Read the model definition and answer for the solid it produces. Units are mm, in the model's axes. A direction names the side the tool comes from. Round coordinates to 2 decimals unless told otherwise and drop trailing zeros. Order: outer loops, then holes, each group sorted by start corner. A loop starts at its lowest first (then second) coordinate and runs counter-clockwise, first axis right, second up. Notation, with made-up numbers: (-34, 73.25) - (-20, 73.25) arc R9 cw to (-20, 80.25) - close; hole circle Ø10 at (-26, 64). An arc over 180 degrees is marked (long way). Answer as a JSON object with one key per item and string values. Group by question number.
Q1. A cutting plane is placed at D-D on z = -27.5. Determine the outline of the cut face in (x, y), and give its area (3 significant figures).
Q2. A tool of negligible diameter and unlimited length cuts with its end or side. For faces 4 (the flat face through (0, 47, -12.5)), 5 (the cylindrical face through (1.352, 22.185, -4.292)), 6 (the flat face through (-12.5, 47, 0)), 7 (the flat face through (3, 51, 0)), from which of +Z, -Z, +X, -X, +Y, -Y can it reach the whole face along a straight path? Write none if from no direction.
Q3. The mould has two halves that part along X. Classify faces 1 (the cylindrical face through (1.43, 21.76, 32.03)), 2 (the flat face through (12.5, 47, 0)), 3 (the flat face through (-9, 0, -1)): pulls with the +X half, pulls with the -X half, needs draft (parallel to the pull), parting line crosses it, or undercut.
Q4. A cutting plane is placed at B-B on y = 42. Determine the outline of the cut face in (x, z), and give its area (3 significant figures).
Q5. A cutting plane is placed at A-A on z = -13.75. Determine the outline of the cut face in (x, y), and give its area (3 significant figures).
Q6. Consider line 1 (Z direction, x = 2.5, y = 37); line 2 (X direction, y = 1.45, z = 13.75); line 3 (Z direction, x = 24, y = 13). Determine where each line is inside the solid, lowest interval first.
Q7. Given pin 1 Ø5 at (x, z) = (-1.5, 27) entering from +Y; pin 2 Ø14.5 at (x, z) = (0, 0) entering from +Y; pin 3 Ø2 at (y, z) = (13.5, -31) entering from +X; pin 4 Ø12 at (y, z) = (31, 9.5) entering from -X, each flat-ended and moving along its own axis, determine where each tip first touches the part or whether it passes through.
Q8. A cutting plane is placed at C-C on x = 0. Count the separate pieces of the cut face and the enclosed holes in it, and give its area (3 significant figures).
```python
from build123d import *

# Parameters (mm, degrees)
SKETCH1_R             = 41.5
MAIN_PLATE_DEPTH      = 40
SKETCH2_R             = 2.05
CUT_EXTRUDE_G27_DEPTH = 72.024643611
SKETCH5_R             = 4.75
G27_SCREW_HEADS_DEPTH = 37
SKETCH6_W             = 25
SKETCH6_H             = 25
BOSS_EXTRUDE1_DEPTH   = 15
SKETCH8_R             = 4.5
CUT_EXTRUDE1_DEPTH    = 45
SKETCH10_R            = 2.5
CUT_EXTRUDE3_DEPTH    = 81.4332021
CUT_EXTRUDE4_DEPTH    = 4


with BuildPart() as part:
    # Sketch1 → Main Plate (new body)
    with BuildSketch(Plane(origin=(0, 0, 0), x_dir=(1, 0, 0), z_dir=(0, 1, 0))):
        with Locations(Location((0, 0, 0), (0, 0, 270))):
            Circle(SKETCH1_R)
    extrude(amount=MAIN_PLATE_DEPTH)

    # Sketch2 → Cut-Extrude G27 (cut, through all)
    with BuildSketch(Plane(origin=(0, 40, 0), x_dir=(1, 0, 0), z_dir=(0, 1, 0))):
        with Locations(Location((0, 27.5, 0), (0, 0, 270))):
            Circle(SKETCH2_R)
        with Locations(Location((23.815698604, 13.75, 0), (0, 0, 270))):
            Circle(SKETCH2_R)
        with Locations(Location((23.815698604, -13.75, 0), (0, 0, 270))):
            Circle(SKETCH2_R)
        with Locations(Location((0, -27.5, 0), (0, 0, 270))):
            Circle(SKETCH2_R)
        with Locations(Location((-23.815698604, -13.75, 0), (0, 0, 270))):
            Circle(SKETCH2_R)
        with Locations(Location((-23.815698604, 13.75, 0), (0, 0, 270))):
            Circle(SKETCH2_R)
    extrude(amount=-CUT_EXTRUDE_G27_DEPTH, mode=Mode.SUBTRACT)

    # Sketch5 → G27 Screw Heads (cut)
    with BuildSketch(Plane(origin=(0, 40, 0), x_dir=(1, 0, 0), z_dir=(0, 1, 0))):
        with Locations(Location((0, 27.5, 0), (0, 0, 270))):
            Circle(SKETCH5_R)
        with Locations(Location((23.815698604, 13.75, 0), (0, 0, 270))):
            Circle(SKETCH5_R)
        with Locations(Location((23.815698604, -13.75, 0), (0, 0, 270))):
            Circle(SKETCH5_R)
        with Locations(Location((0, -27.5, 0), (0, 0, 270))):
            Circle(SKETCH5_R)
        with Locations(Location((-23.815698604, -13.75, 0), (0, 0, 270))):
            Circle(SKETCH5_R)
        with Locations(Location((-23.815698604, 13.75, 0), (0, 0, 270))):
            Circle(SKETCH5_R)
    extrude(amount=-G27_SCREW_HEADS_DEPTH, mode=Mode.SUBTRACT)

    # Sketch6 → Boss-Extrude1 (add)
    with BuildSketch(Plane(origin=(0, 40, 0), x_dir=(1, 0, 0), z_dir=(0, 1, 0))):
        Rectangle(SKETCH6_W, SKETCH6_H)
    extrude(amount=BOSS_EXTRUDE1_DEPTH)

    # Sketch8 → Cut-Extrude1 (cut)
    with BuildSketch(Plane.XZ):
        with Locations(Location((0, 0, 0), (0, 0, 270))):
            Circle(SKETCH8_R)
    extrude(amount=-CUT_EXTRUDE1_DEPTH, mode=Mode.SUBTRACT)

    # Cut-Extrude2 cone 1 section (through the dimple's axis) → Cut-Extrude2 (revolve, cut)
    with BuildSketch(Plane(origin=(0, 45, 0), x_dir=(0, 0, -1), z_dir=(1, 0, 0))):
        Polygon((0, 0), (4.5, 0), (0, 4.5), align=None)
    revolve(axis=Axis((0, 45, 0), (0, 1, 0)), mode=Mode.SUBTRACT)

    # Sketch10 → Cut-Extrude3 (cut, through all)
    with BuildSketch(Plane(origin=(0, 55, 0), x_dir=(1, 0, 0), z_dir=(0, 1, 0))):
        with Locations(Location((0, 0, 0), (0, 0, 270))):
            Circle(SKETCH10_R)
    extrude(amount=-CUT_EXTRUDE3_DEPTH, mode=Mode.SUBTRACT)

    # Sketch11 → Cut-Extrude4 (cut)
    with BuildSketch(Plane(origin=(0, 55, 0), x_dir=(1, 0, 0), z_dir=(0, 1, 0))):
        Polygon((-4.099186911, 0), (-2.049593456, -3.55), (2.049593456, -3.55), (4.099186911, 0), (2.049593456, 3.55), (-2.049593456, 3.55), align=None)
    extrude(amount=-CUT_EXTRUDE4_DEPTH, mode=Mode.SUBTRACT)


solid = part.part
```
Result set:
{
 "1": {"outline": "(-31.08, 0) - (-2.05, 0) - (-2.05, 3) - (-4.75, 3) - (-4.75, 40) - (-31.08, 40) - close; (2.05, 0) - (31.08, 0) - (31.08, 40) - (4.75, 40) - (4.75, 3) - (2.05, 3) - close", "area": "2,120 mm²"},
 "2": {"face 4": "-Z, +X, -X, +Y", "face 5": "-Y", "face 6": "+Z, -Z, -X, +Y", "face 7": "+Y"},
 "3": {"face 1": "undercut", "face 2": "pulls with the +X half", "face 3": "needs draft"},
 "4": {"outline": "(-12.5, -12.5) - (12.5, -12.5) - (12.5, 12.5) - (-12.5, 12.5) - close; hole circle Ø9 at (0, 0)", "area": "561 mm²"},
 "5": {"outline": "(-39.16, 0) - (-25.87, 0) - (-25.87, 3) - (-28.57, 3) - (-28.57, 40) - (-39.16, 40) - close; (-21.77, 0) - (21.77, 0) - (21.77, 3) - (19.07, 3) - (19.07, 40) - (-19.07, 40) - (-19.07, 3) - (-21.77, 3) - close; (25.87, 0) - (39.16, 0) - (39.16, 40) - (28.57, 40) - (28.57, 3) - (25.87, 3) - close", "area": "2,400 mm²"},
 "6": {"line 1": "z = -41.42 to -31.54, -23.46 to -3.74, 3.74 to 23.46, 31.54 to 41.42", "line 2": "x = -39.16 to -25.87, -21.77 to 21.77, 25.87 to 39.16", "line 3": "z = -33.86 to -18.5, -9 to 9, 18.5 to 33.86"},
 "7": {"pin 1": "stops at y = 3", "pin 2": "stops at y = 55", "pin 3": "stops at x = 28.67", "pin 4": "stops at x = -41.35"},
 "8": {"separate pieces": "4", "enclosed holes": "0", "area": "2,500 mm²"}
}
